Could you check a few things on this model? Use its own coordinates, in mm. A direction names the side the tool comes from. Round coordinates to 2 decimals unless told otherwise and drop trailing zeros. Loops run counter-clockwise (first coordinate to the right, second up) from the corner with the lowest first, then second, coordinate; pieces in that order, holes last.
Autodesk Inventor part; units mm, degrees
ref_plane "YZ Plane" through (0, 0, 0) normal (1, 0, 0) x (0, 1, 0)
ref_plane "XZ Plane" through (0, 0, 0) normal (0, 1, 0) x (-1, 0, 0)
ref_plane "XY Plane" through (0, 0, 0) normal (0, 0, 1) x (1, 0, 0)
sketch "Sketch1" plane through (0, 0, 0) normal (0, 1, 0) x (-1, 0, 0)
  line L0 (7, -7.5) -> (-7, -7.5)
  line L1 (-7, -7.5) -> (-7, 7.5)
  line L2 (7, 7.5) -> (7, -7.5)
  line L3 (9.5, -10) -> (-9.5, -10)
  line L4 (9.5, 7.5) -> (9.5, -10)
  line L5 (7, 7.5) -> (9.5, 7.5)
  line L6 (-7, 7.5) -> (-9.5, 7.5)
  line L7 (-9.5, 7.5) -> (-9.5, -10)
  point P0 (0, 0)
  point P1 (0, -7.5)
  point P2 (7, 0)
  point P3 (9.5, 0)
  point P4 (0, -10)
  point P5 (8.25, 7.5)
  point P6 (-8.25, 7.5)
  dimension "d0" = 14
  dimension "d1" = 15
  dimension "d2" = 19
  dimension "d4" = 2.5
extrude "Extrusion1" add sketch "Sketch1" along normal blind 10
sketch "Sketch2" plane through (-7, 0, -7.5) normal (0, 0, 1) x (1, 0, 0)
  point P0 (7, 0)
sketch "Sketch3" plane through (-7, 0, -7.5) normal (0, 0, 1) x (1, 0, 0)
  line L0 (0, 0) -> (14, 0)
  line L1 (14, 0) -> (14, 10)
  point P0 (7, 0)
  point P1 (10.5, 5)
  point P2 (3.5, 5)
  point P3 (7, 5)
  point P4 (7, 0)
  point P5 (14, 5)
  point P6 (7, 0)
  point P7 (7, 0)
  point P8 (14, 5)
  dimension "d7" = 7
  dimension "d8" = 3.5
  dimension "d9" = 3.5
hole "Hole1" at (-3.5, 5, -7.5) at (3.5, 5, -7.5) direction (0, 0, -1) diameter 3 depth 2.5
sketch "Sketch4" plane through (9.5, 0, 7.5) normal (1, 0, 0) x (0, 0, -1)
  line L0 (17.5, 0) -> (17.5, 10)
  point P0 (7.5, 0)
  point P1 (5.5, 5)
  point P2 (15, 10)
  point P3 (17.5, 5)
  dimension "d21" = 9.5
hole "Hole2" at (9.5, 5, 2) direction (-1, 0, 0) diameter 3 depth 19
fillet "Fillet1" radius 1 10 edges at (9.5, 10, -1.25) (9.5, 0, -1.25) (9.5, 5, 7.5) (9.5, 5, -10) (0, 10, -10) (0, 0, -10) (-9.5, 5, -10) (-9.5, 10, -1.25) (-9.5, 0, -1.25) (-9.5, 5, 7.5)
properties part number "Part_B6"
Item 1: If we section it at B-B, the plane y = 5: Please give me the cut outline in (x, z).
Results list:
outline: (-9.5, -9) arc R1 ccw to (-8.5, -10) - (-5, -10) - (-5, -7.5) - (-7, -7.5) - (-7, 0.5) - (-9.5, 0.5) - close; (-9.5, 3.5) - (-7, 3.5) - (-7, 7.5) - (-8.5, 7.5) arc R1 ccw to (-9.5, 6.5) - close; (-2, -10) - (2, -10) - (2, -7.5) - (-2, -7.5) - close; (5, -10) - (8.5, -10) arc R1 ccw to (9.5, -9) - (9.5, 0.5) - (7, 0.5) - (7, -7.5) - (5, -7.5) - close; (7, 3.5) - (9.5, 3.5) - (9.5, 6.5) arc R1 ccw to (8.5, 7.5) - (7, 7.5) - close
Item 2: For faces 1 (the flat face through (-9.5, 5, -1)), 2 (the flat face through (0, 5, -7.5)), which set-ups out of +Z, -Z, +X, -X, +Y, -Y let a thin tool reach every point of the face, with its end or its side?
Results list:
face 1: +Z, -Z, -X, +Y, -Y
face 2: +Z, +Y, -Y
Item 3: If I drill on line 1 along X through (y, z) = (5.5, -2.5); line 2 along Y through (x, z) = (-7.9, 2); line 3 along X through (y, z) = (5, -8.4), over which ranges is the centre line in solid material (lowest first)?
Results list:
line 1: x = -9.5 to -7, 7 to 9.5
line 2: y = 0 to 3.5, 6.5 to 10
line 3: x = -9.5 to -5, -2 to 2, 5 to 9.5
Item 4: If we section it at A-A, the plane z = -2.5: Please give me the cut outline in (x, y).
Results list:
outline: (-9.5, 1) arc R1 ccw to (-8.5, 0) - (-7, 0) - (-7, 10) - (-8.5, 10) arc R1 ccw to (-9.5, 9) - close; (7, 0) - (8.5, 0) arc R1 ccw to (9.5, 1) - (9.5, 9) arc R1 ccw to (8.5, 10) - (7, 10) - close
Item 5: Will these pins go through, and if not, where does the flat tip stop? pin 1 (6 mm diameter, centred on x = 0, z = -2.5, fed in from +Y); pin 2 (4 mm diameter, centred on x = 3.5, y = 5, fed in from +Z).
Results list:
pin 1: passes through
pin 2: stops at z = -7.5
Item 6: If we section it at C-C, the plane x = -3.5: Please give me the cut outline in (y, z).
Results list:
outline: (0, -9) arc R1 ccw to (1, -10) - (3.5, -10) - (3.5, -7.5) - (0, -7.5) - close; (6.5, -10) - (9, -10) arc R1 ccw to (10, -9) - (10, -7.5) - (6.5, -7.5) - close
Item 7: If we section it at D-D, the plane z = 2: Please give me the cut outline in (x, y).
Results list:
outline: (-9.5, 1) arc R1 ccw to (-8.5, 0) - (-7, 0) - (-7, 3.5) - (-9.5, 3.5) - close; (-9.5, 6.5) - (-7, 6.5) - (-7, 10) - (-8.5, 10) arc R1 ccw to (-9.5, 9) - close; (7, 0) - (8.5, 0) arc R1 ccw to (9.5, 1) - (9.5, 3.5) - (7, 3.5) - close; (7, 6.5) - (9.5, 6.5) - (9.5, 9) arc R1 ccw to (8.5, 10) - (7, 10) - close
Item 8: We'd pull the mould along Y, two halves only. Please class faces 3 (the cylindrical face through (2.49, 6.11, -8.77)), 4 (the cylindrical face through (9.199, 9.715, -0.865)), 5 (the cylindrical face through (-2.6, 6.2, -8.8)), 6 (the cylindrical face through (9.199, 5.07, 7.215)): released by +Y, released by -Y, zero draft, split by the parting line, or undercut.
Results list:
face 3: undercut
face 4: released by +Y
face 5: undercut
face 6: zero draft
